Source: CAD feature listing. Evaluate the final solid. Frame: model axes, mm. Face numbers are marked on the shaded views. A direction names the side the tool comes from. Coordinates: 2 decimals unless noted, no trailing zeros. Order: outer loops, then holes, each group sorted by start corner. A loop starts at its lowest first (then second) coordinate and runs counter-clockwise, first axis right, second up. Notation, with made-up numbers: (70, 70.5) - (108, 70.5) arc R19 cw to (108, 94.5) - close; hole circle Ø4 at (5, 53.5). An arc over 180 degrees is marked (long way). One line per question, with ' | ' between items. Start each with the question number.
(1) Access query for the marked faces 1 and 2. Directions: +Z, -Z, +X, -X, +Y, -Y. A direction counts if a zero-diameter tool reaches every point of the face in a straight line with its end or side. Return the directions, or none.
(2) Section B-B (x = -4.5). Return the cut outline in (y, z).
(3) Section C-C (y = 2.25). Return the cut outline in (x, z), then the cut area to 3 significant figures.
(4) Contact query for flat-ended pins moving along their axis: P1, Ø4, axis at x = -0.5, y = 6, coming from the +Z side; P2, Ø1, axis at y = 10, z = -5, coming from the +X side; P3, Ø1.5, axis at y = 5, z = -4.5, coming from the +X side; P4, Ø4, axis at x = -5, z = -2, coming from the -Y side. Output: stop coordinate, or through.
(5) Line query: line 1 along Y through (x, z) = (-4, -3.25); line 2 along X through (y, z) = (1.5, -4.75); line 3 along X through (y, z) = (7.5, -3.75). Output: solid intervals per line, ascending.
(6) Section A-A (z = -2). Return the cut outline in (x, y), then the cut area to 3 significant figures.
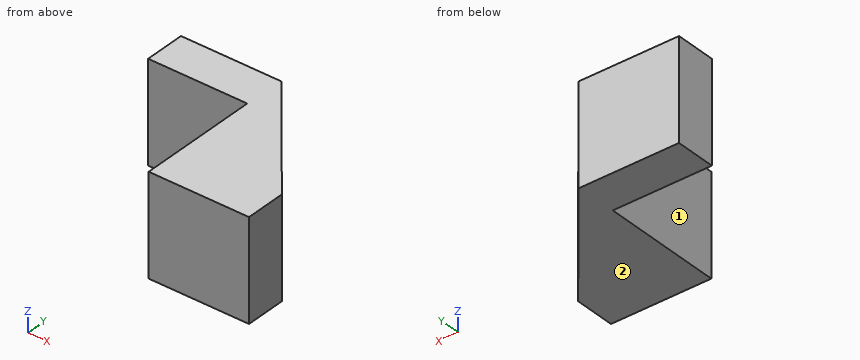
from build123d import *

# Parameters (mm, degrees)
SKETCH1_W           = 7.9
SKETCH1_H           = 7.9
BOSS_EXTRUDE1_DEPTH = 3.2
SKETCH2_W           = 7.9
SKETCH2_H           = 9.6
BOSS_EXTRUDE2_DEPTH = 0.1
SKETCH3_W           = 7.9
SKETCH3_H           = 7.9
BOSS_EXTRUDE3_DEPTH = 3.2
BOSS_EXTRUDE4_DEPTH = 7.9


with BuildPart() as part:
    # Sketch1 → Boss-Extrude1 (new body)
    with BuildSketch(Plane(origin=(0, 0, 0), x_dir=(1, 0, 0), z_dir=(0, 1, 0))):
        with Locations((3.95, 3.95)):
            Rectangle(SKETCH1_W, SKETCH1_H)
    extrude(amount=BOSS_EXTRUDE1_DEPTH)

    # Sketch2 → Boss-Extrude2 (add)
    with BuildSketch(Plane.ZY):
        with Locations((-3.95, 4.8)):
            Rectangle(SKETCH2_W, SKETCH2_H)
    extrude(amount=-BOSS_EXTRUDE2_DEPTH)

    # Sketch3 → Boss-Extrude3 (add)
    with BuildSketch(Plane(origin=(0, 9.6, 0), x_dir=(1, 0, 0), z_dir=(0, 1, 0))):
        with Locations((-3.85, 3.95)):
            Rectangle(SKETCH3_W, SKETCH3_H)
    extrude(amount=BOSS_EXTRUDE3_DEPTH)

    # Sketch4 → Boss-Extrude4 (add)
    with BuildSketch(Plane.XY):
        Polygon((0.1, 12.8), (7.9, 3.2), (0.1, 3.2), align=None)
    extrude(amount=-BOSS_EXTRUDE4_DEPTH)


solid = part.part
Response values:
1) face 1: +Z, -Z, -X, -Y | face 2: -Z, +X, -X, +Y, -Y
2) outline: (9.6, -7.9) - (12.8, -7.9) - (12.8, 0) - (9.6, 0) - close
3) outline: (0, -7.9) - (7.9, -7.9) - (7.9, 0) - (0, 0) - close | area: 62.4 mm²
4) P1: stops at z = 0 | P2: stops at x = 2.78 | P3: stops at x = 7.05 | P4: stops at y = 9.6
5) line 1: y = 9.6 to 12.8 | line 2: x = 0 to 7.9 | line 3: x = 0 to 4.41
6) outline: (-7.8, 9.6) - (0, 9.6) - (0, 0) - (7.9, 0) - (7.9, 3.2) - (0.1, 12.8) - (-7.8, 12.8) - close | area: 88.6 mm²
